Here's how the part is built. I have some questions about the finished solid (model axes, mm). A direction names the side the tool comes from. Round coordinates to 2 decimals unless told otherwise and drop trailing zeros. Order: outer loops, then holes, each group sorted by start corner. A loop starts at its lowest first (then second) coordinate and runs counter-clockwise, first axis right, second up. Notation, with made-up numbers: M 89.5,65.25 L 96.5,65.25 A14 ccw 96.5,77.25 Z; hole C 2.25,-33.75 d7. An arc over 180 degrees is marked long. Answer as CSV lines item,"result". Start each with the question number.
```python
from build123d import *

# Parameters (mm, degrees)
PAD_DEPTH       = 3
SKETCH001_R     = 9.7
PAD001_DEPTH    = 5
SKETCH002_R     = 4.5
POCKET_DEPTH    = 8.001
POCKET001_DEPTH = 5
FILLET_R        = 1
FILLET001_R     = 2.49


with BuildPart() as part:
    # Sketch → Pad (new body)
    with BuildSketch(Plane.XY):
        with BuildLine():
            ThreePointArc((12.247449, 2.5), (0, 12.5), (-12.247449, 2.5))
            Line((-12.247449, 2.5), (-17.247449, 2.5))
            Line((-17.247449, 2.5), (-17.247449, -2.5))
            Line((-17.247449, -2.5), (-12.247449, -2.5))
            ThreePointArc((-12.247449, -2.5), (0, -12.5), (12.247449, -2.5))
            Line((17.247449, -2.5), (12.247449, -2.5))
            Line((17.247449, 2.5), (17.247449, -2.5))
            Line((12.247449, 2.5), (17.247449, 2.5))
        make_face()
    extrude(amount=PAD_DEPTH)

    # Sketch001 → Pad001 (new body)
    with BuildSketch(Plane.XY.offset(3)):
        Circle(SKETCH001_R)
    extrude(amount=PAD001_DEPTH)

    # Sketch002 → Pocket (cut, through all)
    with BuildSketch(Plane.XY.offset(8)):
        Circle(SKETCH002_R)
    extrude(amount=-POCKET_DEPTH, mode=Mode.SUBTRACT)

    # Sketch003 → Pocket001 (cut)
    with BuildSketch(Plane(origin=(0, 0, 0), x_dir=(1, 0, 0), z_dir=(0, 0, -1))):
        Polygon((3.810512, -6.6), (7.621024, 0), (3.810512, 6.6), (-3.810512, 6.6), (-7.621024, 0), (-3.810512, -6.6), align=None)
    extrude(amount=-POCKET001_DEPTH, mode=Mode.SUBTRACT)

    # Fillet
    fillet_edges = [part.edges().sort_by_distance(p)[0] for p in [
        (-9.7, 0, 8),
    ]]
    fillet(fillet_edges, radius=FILLET_R)

    # Fillet001
    fillet001_edges = [part.edges().sort_by_distance(p)[0] for p in [
        (12.247449, 2.5, 1.5),
        (17.247449, 2.5, 1.5),
        (17.247449, -2.5, 1.5),
        (12.247449, -2.5, 1.5),
        (-12.247449, -2.5, 1.5),
        (-17.247449, -2.5, 1.5),
        (-17.247449, 2.5, 1.5),
        (-12.247449, 2.5, 1.5),
    ]]
    fillet(fillet001_edges, radius=FILLET001_R)


solid = part.part
```
Item 1: If we section it at C-C on z = 6: Please give me the cut outline in (x, y).
Item 2: If we section it at A-A on x = 0: Please give me the cut outline in (y, z), and give its area (3 significant figures).
Item 3: Which directions (+Z, -Z, +X, -X, +Y, -Y) give clear straight access to the entire face, cutting with the end or side of a thin tool? Please do faces 1 (the flat face through (-5.689, -3.346, 2.465)), 2 (the cylindrical face through (9.252, 2.914, 4.972)), 3 (the cylindrical face through (12.715, -2.945, 1.521)).
Item 4: If I drill on line 1 along Y through (x, z) = (0, 6.5); line 2 along Z through (x, y) = (-3, 4); line 3 along Z through (x, y) = (7, -5.25), over which ranges is the centre line in solid material (lowest first)?
Item 5: We'd pull the mould along Y, two halves only. Please class faces 4 (the cylindrical face through (16.54, -1.75, 1.52)), 5 (the cylindrical face through (-12.68, 2.97, 1.52)), 6 (the flat face through (0, -6.6, 2)): pulls with the +Y half, pulls with the -Y half, needs draft (parallel to the pull), parting line crosses it, or undercut.
Item 6: For P1, Ø0.7, axis at x = -14.5, z = 1, coming from the +Y side; P2, Ø3, axis at x = -2, z = 5.5, coming from the -Y side; P3, Ø8, axis at x = -9.5, y = -7.5, coming from the -Z side; P4, Ø2, axis at y = -3.5, z = 6, coming from the +X side, each with a flat end and sliding along its axis, tell me the tip position at first contact or that it passes through.
Geometry says:
1,outline,"C 0,0 d19.4; hole C 0,0 d9"
2,outline,"M -12.5,0 L -6.6,0 L -6.6,5 L -4.5,5 L -4.5,8 L -8.7,8 A1 ccw -9.7,7 L -9.7,3 L -12.5,3 Z; M 4.5,5 L 6.6,5 L 6.6,0 L 12.5,0 L 12.5,3 L 9.7,3 L 9.7,7 A1 ccw 8.7,8 L 4.5,8 Z"
2,area,"78.6 mm²"
3,face 1,"-Z"
3,face 2,"+Z"
3,face 3,"+Z, -Z, +X, -Y"
4,line 1,"-9.7 to -4.5, 4.5 to 9.7"
4,line 2,"5 to 8"
4,line 3,"0 to 8"
5,face 4,"pulls with the -Y half"
5,face 5,"pulls with the +Y half"
5,face 6,"undercut"
6,P1,"y = 2.5"
6,P2,"y = -9.69"
6,P3,"z = 0"
6,P4,"x = 9.37"
